Work out the finished part from the listing and answer in its coordinate system (mm). A direction names the side the tool comes from. Coordinates: 2 decimals unless noted, no trailing zeros. Write each loop counter-clockwise with the first axis right and the second up, starting at its lowest first coordinate (ties: lowest second). Pieces come first, ordered by that corner, then holes. Notation, with made-up numbers: (84.5, -36.75) - (131.5, -36.75) arc R25 ccw to (131.5, -7.75) - close; hole circle Ø11 at (-16.75, 34.25). An arc over 180 degrees is marked (long way). One line per item, written item: value.
```python
from build123d import *

# Parameters (mm, degrees)
SKETCH_1_R      = 1.6
EXTRUDE_1_DEPTH = 3
FILLET_1_R      = 2
FILLET_2_R      = 5


with BuildPart() as part:
    # 草图1 → 凸台-拉伸1 (new body)
    with BuildSketch(Plane(origin=(0, 0, 0), x_dir=(1, 0, 0), z_dir=(0, 1, 0))):
        Polygon((0, -45), (-15, -45), (-15, 15), (45, 15), (45, 0), align=None)
        with Locations(Location((-7.5, -12.5, 0), (0, 0, 270))):
            Circle(SKETCH_1_R, mode=Mode.SUBTRACT)
        with Locations(Location((-7.5, -32.5, 0), (0, 0, 270))):
            Circle(SKETCH_1_R, mode=Mode.SUBTRACT)
        with Locations(Location((-7.5, 7.5, 0), (0, 0, 270))):
            Circle(SKETCH_1_R, mode=Mode.SUBTRACT)
        with Locations(Location((12.5, 7.5, 0), (0, 0, 270))):
            Circle(SKETCH_1_R, mode=Mode.SUBTRACT)
        with Locations(Location((32.5, 7.5, 0), (0, 0, 270))):
            Circle(SKETCH_1_R, mode=Mode.SUBTRACT)
        Polygon((0, -33.686291501), (0, 0), (33.686291501, 0), align=None, mode=Mode.SUBTRACT)
    extrude(amount=EXTRUDE_1_DEPTH)

    # 圆角1
    fillet_1_edges = [part.edges().sort_by_distance(p)[0] for p in [
        (0, 1.5, 45),
        (-15, 1.5, 45),
        (-15, 1.5, -15),
        (45, 1.5, -15),
        (45, 1.5, 0),
    ]]
    fillet(fillet_1_edges, radius=FILLET_1_R)

    # 圆角2
    fillet_2_edges = [part.edges().sort_by_distance(p)[0] for p in [
        (33.686291501, 1.5, 0),
        (0, 1.5, 0),
        (0, 1.5, 33.686291501),
    ]]
    fillet(fillet_2_edges, radius=FILLET_2_R)


solid = part.part
```
Item 1: Given pin 1 (2.5 mm diameter, centred on x = -7.5, z = -7.5, fed in from +Y); pin 2 (1.5 mm diameter, centred on y = 2, z = 10.5, fed in from +X), each flat-ended and moving along its own axis, determine where each tip first touches the part or whether it passes through.
Evaluation:
pin 1: passes through
pin 2: stops at x = 35.25
Item 2: Section A-A, the plane z = -7.5 is taken. Determine the outline of the cut face in (x, y).
Evaluation:
outline: (-15, 0) - (-9.1, 0) - (-9.1, 3) - (-15, 3) - close; (-5.9, 0) - (10.9, 0) - (10.9, 3) - (-5.9, 3) - close; (14.1, 0) - (30.9, 0) - (30.9, 3) - (14.1, 3) - close; (34.1, 0) - (45, 0) - (45, 3) - (34.1, 3) - close
Item 3: Determine the mould class of faces 3 (the face through (44.844, 1.521, -0.053)), 4 (the face through (16.959, 1.479, 16.727)), 5 (the face through (22, 0, 15)) for opening direction X: +X half, -X half, draft (parallel to the pull), parting line (faces both ways), or undercut.
Evaluation:
face 3: +X half
face 4: undercut
face 5: draft
Item 4: Which of the six approach directions +Z, -Z, +X, -X, +Y, -Y give full straight-line access (tool end or side, diameter ignored) to faces 1 (the face through (13, 1, 0)), 2 (the face through (-14.4, 1.52, 44.43))?
Evaluation:
face 1: +Y, -Y
face 2: +Z, -X, +Y, -Y
Item 5: Consider probe 1 along X at (y, z) = (2.25, -7.5); probe 2 along X at (y, z) = (2.45, 12.5); probe 3 along Z at (x, y) = (7, 0.2). Determine where each line is inside the solid, lowest interval first.
Evaluation:
probe 1: x = -15 to -9.1, -5.9 to 10.9, 14.1 to 30.9, 34.1 to 45
probe 2: x = -15 to -9.1, -5.9 to 0, 21.19 to 32.5
probe 3: z = -15 to 0, 26.2 to 38
Item 6: Section B-B, the plane x = -7.5 is taken. Determine the outline of the cut face in (y, z).
Evaluation:
outline: (0, -15) - (3, -15) - (3, -9.1) - (0, -9.1) - close; (0, -5.9) - (3, -5.9) - (3, 10.9) - (0, 10.9) - close; (0, 14.1) - (3, 14.1) - (3, 30.9) - (0, 30.9) - close; (0, 34.1) - (3, 34.1) - (3, 45) - (0, 45) - close
Item 7: Section C-C, the plane y = 0.45 is taken. Determine the outline of the cut face in (x, z), then the cut area to 3 significant figures.
Evaluation:
outline: (-15, -13) arc R2 ccw to (-13, -15) - (43, -15) arc R2 ccw to (45, -13) - (45, -0.83) arc R2 ccw to (44.41, 0.59) - (0.59, 44.41) arc R2 ccw to (-0.83, 45) - (-13, 45) arc R2 ccw to (-15, 43) - close; hole circle Ø3.2 at (-7.5, -7.5); hole circle Ø3.2 at (-7.5, 12.5); hole circle Ø3.2 at (-7.5, 32.5); hole (0, 5) arc R5 ccw to (5, 0) - (21.62, 0) arc R5 ccw to (25.15, 8.54) - (8.54, 25.15) arc R5 ccw to (0, 21.62) - close; hole circle Ø3.2 at (12.5, -7.5); hole circle Ø3.2 at (32.5, -7.5)
area: 2,040 mm2
Item 8: Section D-D, the plane x = 32.5 is taken. Determine the outline of the cut face in (y, z), then the cut area to 3 significant figures.
Evaluation:
outline: (0, -15) - (3, -15) - (3, -9.1) - (0, -9.1) - close; (0, -5.9) - (3, -5.9) - (3, 12.5) - (0, 12.5) - close
area: 72.9 mm2
